from build123d import *

# Parameters (mm, degrees)
PAD_DEPTH            = 22
POCKET_DEPTH         = 20
PAD001_DEPTH         = 20
POCKET001_DEPTH      = 5
SKETCH004_R          = 1.5
SKETCH004_W          = 80
SKETCH004_H          = 10
POCKET002_DEPTH      = 78.001
CHAMFER_SIZE         = 5.2
SKETCH005_R          = 15
POCKET003_DEPTH      = 1.2
POCKET004_DEPTH      = 29.001
POCKET004_DEPTH_BACK = -29.001


with BuildPart() as part:
    # Sketch → Pad (new body)
    with BuildSketch(Plane.XY):
        with BuildLine():
            Line((-27, 29), (27, 29))
            ThreePointArc((29, 27), (28.414214, 28.414214), (27, 29))
            Line((29, 27), (29, -27))
            ThreePointArc((27, -29), (28.414214, -28.414214), (29, -27))
            Line((27, -29), (-27, -29))
            ThreePointArc((-29, -27), (-28.414214, -28.414214), (-27, -29))
            Line((-29, -27), (-29, 27))
            ThreePointArc((-27, 29), (-28.414214, 28.414214), (-29, 27))
        make_face()
    extrude(amount=PAD_DEPTH)

    # Sketch001 (on Face10 of Pad) → Pocket (cut)
    with BuildSketch(Plane.XY.offset(22)):
        with BuildLine():
            Line((-18.75, 27.75), (18.75, 27.75))
            Line((18.75, 27.75), (18.75, 26.75))
            ThreePointArc((18.75, 26.75), (21.093146, 21.093146), (26.75, 18.75))
            Line((26.75, 18.75), (27.75, 18.75))
            Line((27.75, 18.75), (27.75, -18.75))
            Line((27.75, -18.75), (26.75, -18.75))
            ThreePointArc((26.75, -18.75), (21.093146, -21.093146), (18.75, -26.75))
            Line((18.75, -26.75), (18.75, -27.75))
            Line((18.75, -27.75), (-18.75, -27.75))
            Line((-18.75, -27.75), (-18.75, -26.75))
            ThreePointArc((-18.75, -26.75), (-21.093146, -21.093146), (-26.75, -18.75))
            Line((-26.75, -18.75), (-27.75, -18.75))
            Line((-27.75, -18.75), (-27.75, 18.75))
            Line((-27.75, 18.75), (-26.75, 18.75))
            ThreePointArc((-26.75, 18.75), (-21.093146, 21.093146), (-18.75, 26.75))
            Line((-18.75, 26.75), (-18.75, 27.75))
        make_face()
    extrude(amount=-POCKET_DEPTH, mode=Mode.SUBTRACT)

    # Sketch002 (on Face1 of Pocket) → Pad001 (join)
    with BuildSketch(Plane(origin=(0, 29, 0), x_dir=(-1, 0, 0), z_dir=(0, 1, 0))):
        with BuildLine():
            ThreePointArc((-6.5, 19.741657), (-10.084682, 12.694582), (-7.5, 5.222592))
            Line((-7.5, 5.222592), (-7.5, 0))
            Line((-7.5, 0), (7.5, 0))
            Line((7.5, 0), (7.5, 5.222592))
            ThreePointArc((7.5, 5.222592), (10.084682, 12.694582), (6.5, 19.741657))
            Line((6.5, 15.741657), (6.5, 19.741657))
            ThreePointArc((-6.5, 15.741657), (0, 4.5), (6.5, 15.741657))
            Line((-6.5, 15.741657), (-6.5, 19.741657))
        make_face()
    extrude(amount=PAD001_DEPTH)

    # Sketch003 → Pocket001 (cut)
    with BuildSketch(Plane(origin=(0, 29, 0), x_dir=(-1, 0, 0), z_dir=(0, 1, 0))):
        with BuildLine():
            ThreePointArc((-6.5, 15.741657), (0, 4.5), (6.5, 15.741657))
            Line((6.5, 25.741657), (6.5, 15.741657))
            Line((-6.5, 25.741657), (6.5, 25.741657))
            Line((-6.5, 15.741657), (-6.5, 25.741657))
        make_face()
    extrude(amount=-POCKET001_DEPTH, mode=Mode.SUBTRACT)

    # Sketch004 → Pocket002 (cut, through all)
    with BuildSketch(Plane.XZ.offset(29)):
        with Locations((-24, 10)):
            Circle(SKETCH004_R)
        with Locations((24, 10)):
            Circle(SKETCH004_R)
        with Locations((0, 22)):
            Rectangle(SKETCH004_W, SKETCH004_H)
    extrude(amount=-POCKET002_DEPTH, mode=Mode.SUBTRACT)

    # Chamfer
    chamfer_edges = [part.edges().sort_by_distance(p)[0] for p in [
        (7.5, 39, 0),
        (-7.5, 39, 0),
    ]]
    chamfer(chamfer_edges, length=CHAMFER_SIZE)

    # Sketch005 (on Face42 of Chamfer) → Pocket003 (cut)
    with BuildSketch(Plane.XY.offset(2)):
        Circle(SKETCH005_R)
    extrude(amount=-POCKET003_DEPTH, mode=Mode.SUBTRACT)

    # Sketch006 → Pocket004 (cut, two sides)
    with BuildSketch(Plane.YZ) as pocket004_sk:
        with BuildLine():
            ThreePointArc((34, 3), (33, 2), (34, 1))
            Line((34, 1), (38, 1))
            ThreePointArc((38, 1), (39, 2), (38, 3))
            Line((34, 3), (38, 3))
        make_face()
        with BuildLine():
            ThreePointArc((42, 3), (41, 2), (42, 1))
            Line((42, 1), (46, 1))
            ThreePointArc((46, 1), (47, 2), (46, 3))
            Line((42, 3), (46, 3))
        make_face()
    extrude(amount=-POCKET004_DEPTH, mode=Mode.SUBTRACT)
    extrude(pocket004_sk.sketch, amount=-POCKET004_DEPTH_BACK, mode=Mode.SUBTRACT)


solid = part.part
Geometry check sheet. Reference: the model listing, model coordinates, mm. A direction names the side the tool comes from. Round coordinates to 2 decimals unless told otherwise and drop trailing zeros. Loops run counter-clockwise (first coordinate to the right, second up) from the corner with the lowest first, then second, coordinate; pieces in that order, holes last. Notation, with made-up numbers: (15.5, 77) - (65.5, 77) arc R29 cw to (65.5, 115) - close; hole circle Ø10 at (15.5, -23.75). An arc over 180 degrees is marked (long way). One line per question, with ' | ' between items. Start each with the question number.
1. Cross-section at A-A on x = 0. Record the cut outline in (y, z).
2. Scan lines: line 1 (Z direction, x = 24, y = -24); line 2 (Z direction, x = 0, y = 44); line 3 (X direction, y = -25.75, z = 10). Record each from-to range of solid material in increasing order. Write a range as [from, to].
3. Cross-section at B-B on x = 17. Record the cut outline in (y, z), then the cut area to 4 significant figures.
4. Draft check along Z on faces 1 (the face through (10.058, 38.86, 10.991)), 2 (the face through (0, 36, 3)), 3 (the face through (29, 0, 8)). Enter one of: released by +Z, released by -Z, zero draft, split by the parting line, or undercut.
5. Depth check by flat-ended pin: pin 1 (2.5 mm diameter, centred on x = 24, z = 10, fed in from +Y); pin 2 (9 mm diameter, centred on x = 5, y = -5.5, fed in from +Z); pin 3 (4 mm diameter, centred on x = -24, z = 10, fed in from +Y); pin 4 (5 mm diameter, centred on y = 40.5, z = 9.5, fed in from -X). Enter the tip coordinate at first touch or a pass-through.
6. Cross-section at C-C on y = 11. Record the cut outline in (x, z).
7. Tool access check on faces 4 (the face through (-21.031, -21.156, 9.605)), 5 (the face through (0, 33, 2)), 6 (the face through (-28.4, 28.43, 8.38)). Record the directions out of +Z, -Z, +X, -X, +Y, -Y that give a thin tool (end or side, any length) a straight path to the whole face; none if there is none.
Taken from the geometry:
1) outline: (-29, 0) - (49, 0) - (49, 4.5) - (27.75, 4.5) - (27.75, 2) - (15, 2) - (15, 0.8) - (-15, 0.8) - (-15, 2) - (-27.75, 2) - (-27.75, 17) - (-29, 17) - close; hole (34, 1) - (38, 1) arc R1 ccw to (38, 3) - (34, 3) arc R1 ccw to start; hole (42, 1) - (46, 1) arc R1 ccw to (46, 3) - (42, 3) arc R1 ccw to start
2) line 1: [0, 8.5], [11.5, 17] | line 2: [0, 1], [3, 4.5] | line 3: [-29, -25.5], [-22.5, -18.81], [18.81, 22.5], [25.5, 29]
3) outline: (-29, 0) - (29, 0) - (29, 17) - (27.75, 17) - (27.75, 2) - (-27.75, 2) - (-27.75, 17) - (-29, 17) - close | area: 153.5 mm²
4) face 1: split by the parting line | face 2: undercut | face 3: zero draft
5) pin 1: through | pin 2: z = 0.8 | pin 3: y = 29 | pin 4: x = -10.11
6) outline: (-29, 0) - (29, 0) - (29, 17) - (27.75, 17) - (27.75, 2) - (10.2, 2) - (10.2, 0.8) - (-10.2, 0.8) - (-10.2, 2) - (-27.75, 2) - (-27.75, 17) - (-29, 17) - close
7) face 4: +Z | face 5: +X, -X | face 6: +Z, -Z, -X, +Y
